Design review of the part shown in the three views and the two pictorial views. Dimensions are in mm from the part's minimum x, y and z. Give positions to 0.01 mm unless a question says otherwise; leave off trailing zeros. Loops run counter-clockwise (first coordinate to the right, second up) from the corner with the lowest first, then second, coordinate; pieces in that order, holes last. Notation, with made-up numbers: (1.5, 7) -> (33.5, 7) arc R24 ccw to (33.5, 28) -> close; hole circle Ø5 at (23.25, 63.5). An arc over 180 degrees is marked (long way). Use CSV: the item, a comma, the result in double quotes. Start each with the question number.
Item 1: Clearance check with a flat-ended pin moving along its axis: pin 1 (4.5 mm diameter, centred on x = 44.25, y = 45.7, fed in from -Z). State where the tip first meets the part, or that it passes through.
Item 2: We need section A-A (x = 44.25). State the section outline as (y, z) points, plus the area to 3 significant figures.
Item 3: Wall thickness on line 1 along Y through (x, z) = (44.25, 1.4): over which ranges is the line inside the solid? List them lowest first. Write a range as from..to.
Item 4: We need section B-B (y = 45.7). State the section outline as (x, z) points.
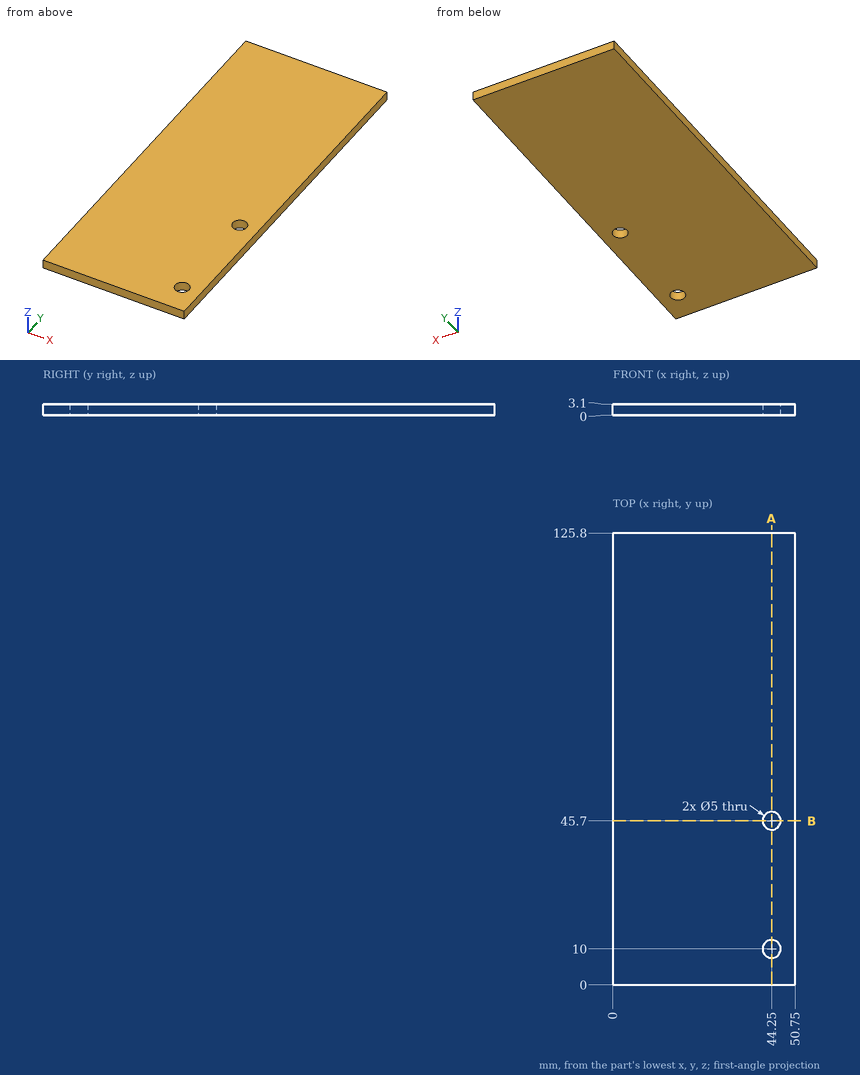
Results found:
1,pin 1,"through"
2,outline,"(0, 0) -> (7.5, 0) -> (7.5, 3.1) -> (0, 3.1) -> close; (12.5, 0) -> (43.2, 0) -> (43.2, 3.1) -> (12.5, 3.1) -> close; (48.2, 0) -> (125.8, 0) -> (125.8, 3.1) -> (48.2, 3.1) -> close"
2,area,"359 mm²"
3,line 1,"0..7.5, 12.5..43.2, 48.2..125.8"
4,outline,"(0, 0) -> (41.75, 0) -> (41.75, 3.1) -> (0, 3.1) -> close; (46.75, 0) -> (50.75, 0) -> (50.75, 3.1) -> (46.75, 3.1) -> close"
